Work out the finished part from the listing and answer in its coordinate system (mm). Round coordinates to 2 decimals unless told otherwise and drop trailing zeros. Loops run counter-clockwise (first coordinate to the right, second up) from the corner with the lowest first, then second, coordinate; pieces in that order, holes last. Notation, with made-up numbers: (42.25, -6) - (69.25, -6) arc R20 ccw to (69.25, 20) - close; hole circle Ø5 at (83, -21). An arc over 180 degrees is marked (long way). Return JSON: item names as keys, results as strings.
from build123d import *

# Parameters (mm, degrees)
MODEL_R         = 1
MODEL_R_2       = 1.5
EXTRUDE_1_DEPTH = 2


with BuildPart() as part:
    # Model → 凸台-拉伸1 (new body)
    with BuildSketch(Plane.XY):
        with BuildLine():
            ThreePointArc((165.794247794, 119.146851779), (174.607099306, 112.447515783), (184.890996066, 108.350087077))
            ThreePointArc((184.890996066, 108.350087077), (190.059733129, 100.139821501), (184.890996066, 91.929555925))
            ThreePointArc((184.890996066, 91.929555925), (174.607099306, 87.832127219), (165.794247794, 81.132791223))
            ThreePointArc((165.794247794, 81.132791223), (159.094911797, 72.319939711), (154.997483091, 62.036042951))
            ThreePointArc((154.997483091, 62.036042951), (146.787217515, 56.867305888), (138.576951939, 62.036042951))
            ThreePointArc((138.576951939, 62.036042951), (134.479523234, 72.319939711), (127.780187237, 81.132791223))
            ThreePointArc((127.780187237, 81.132791223), (118.967335725, 87.832127219), (108.683438965, 91.929555925))
            ThreePointArc((108.683438965, 91.929555925), (103.514701902, 100.139821501), (108.683438965, 108.350087077))
            ThreePointArc((108.683438965, 108.350087077), (118.967335725, 112.447515783), (127.780187237, 119.146851779))
            ThreePointArc((127.780187237, 119.146851779), (134.479523234, 127.959703291), (138.576951939, 138.243600051))
            ThreePointArc((138.576951939, 138.243600051), (146.787217515, 143.412337115), (154.997483091, 138.243600051))
            ThreePointArc((154.997483091, 138.243600051), (159.094911797, 127.959703291), (165.794247794, 119.146851779))
        make_face()
        with Locations((156.787217515, 110.139821501)):
            Circle(MODEL_R, mode=Mode.SUBTRACT)
        with Locations((136.787217515, 110.139821501)):
            Circle(MODEL_R, mode=Mode.SUBTRACT)
        with Locations((136.787217515, 90.139821501)):
            Circle(MODEL_R, mode=Mode.SUBTRACT)
        with Locations((156.787217515, 90.139821501)):
            Circle(MODEL_R, mode=Mode.SUBTRACT)
        with Locations((168.353974342, 100.139821501)):
            Circle(MODEL_R_2, mode=Mode.SUBTRACT)
        with Locations((146.787217515, 121.706578327)):
            Circle(MODEL_R_2, mode=Mode.SUBTRACT)
        with Locations((125.220460689, 100.139821501)):
            Circle(MODEL_R_2, mode=Mode.SUBTRACT)
        with Locations((146.787217515, 78.573064675)):
            Circle(MODEL_R_2, mode=Mode.SUBTRACT)
        with Locations((146.787217515, 126.706578327)):
            Circle(MODEL_R_2, mode=Mode.SUBTRACT)
        with Locations((120.220460689, 100.139821501)):
            Circle(MODEL_R_2, mode=Mode.SUBTRACT)
        with Locations((146.787217515, 73.573064675)):
            Circle(MODEL_R_2, mode=Mode.SUBTRACT)
        with Locations((173.353974342, 100.139821501)):
            Circle(MODEL_R_2, mode=Mode.SUBTRACT)
        with Locations((146.787217515, 118.171044401)):
            Circle(MODEL_R, mode=Mode.SUBTRACT)
        with Locations((128.755994615, 100.139821501)):
            Circle(MODEL_R, mode=Mode.SUBTRACT)
        with Locations((146.787217515, 82.108598601)):
            Circle(MODEL_R, mode=Mode.SUBTRACT)
        with Locations((164.818440415, 100.139821501)):
            Circle(MODEL_R, mode=Mode.SUBTRACT)
        with Locations((162.037217515, 115.389821501)):
            Circle(MODEL_R_2, mode=Mode.SUBTRACT)
        with Locations((131.537217515, 115.389821501)):
            Circle(MODEL_R_2, mode=Mode.SUBTRACT)
        with Locations((131.537217515, 84.889821501)):
            Circle(MODEL_R_2, mode=Mode.SUBTRACT)
        with Locations((162.037217515, 84.889821501)):
            Circle(MODEL_R_2, mode=Mode.SUBTRACT)
        with Locations((182.657217515, 100.139821501)):
            Circle(MODEL_R, mode=Mode.SUBTRACT)
        with Locations((146.787217515, 136.036864466)):
            Circle(MODEL_R, mode=Mode.SUBTRACT)
        with Locations((110.917217515, 100.139821501)):
            Circle(MODEL_R, mode=Mode.SUBTRACT)
        with Locations((146.787217515, 64.242778536)):
            Circle(MODEL_R, mode=Mode.SUBTRACT)
        with BuildLine():
            Line((152.398515146, 91.006916148), (141.004728844, 91.006916149))
            ThreePointArc((141.004728844, 91.006916149), (140.104214379, 91.379921453), (139.731209075, 92.280435918))
            ThreePointArc((139.731209075, 92.280435918), (140.104214379, 93.180950383), (141.004728844, 93.553955688))
            Line((141.004728844, 93.553955688), (152.398515146, 93.553955687))
            ThreePointArc((152.398515146, 93.553955687), (153.672034916, 92.280435917), (152.398515146, 91.006916148))
        make_face(mode=Mode.SUBTRACT)
        with BuildLine():
            Line((152.599718137, 109.199272945), (141.205931835, 109.199272945))
            ThreePointArc((141.205931835, 109.199272945), (140.30541737, 108.826267641), (139.932412066, 107.925753176))
            ThreePointArc((139.932412066, 107.925753176), (140.30541737, 107.025238711), (141.205931835, 106.652233406))
            Line((141.205931835, 106.652233406), (152.599718137, 106.652233406))
            ThreePointArc((152.599718137, 106.652233406), (153.873237907, 107.925753176), (152.599718137, 109.199272945))
        make_face(mode=Mode.SUBTRACT)
        with BuildLine():
            Line((151.898560909, 100.493374892), (147.140770906, 105.251164895))
            ThreePointArc((147.140770906, 105.251164895), (146.787217515, 105.397611504), (146.433664125, 105.251164895))
            Line((146.433664125, 105.251164895), (141.675874122, 100.493374892))
            ThreePointArc((141.675874122, 100.493374892), (141.529427512, 100.139821501), (141.675874122, 99.786268111))
            Line((141.675874122, 99.786268111), (146.433664125, 95.028478108))
            ThreePointArc((146.433664125, 95.028478108), (146.787217515, 94.882031498), (147.140770906, 95.028478108))
            Line((147.140770906, 95.028478108), (151.898560909, 99.786268111))
            ThreePointArc((151.898560909, 99.786268111), (152.045007518, 100.139821501), (151.898560909, 100.493374892))
        make_face(mode=Mode.SUBTRACT)
        with BuildLine():
            Line((137.779884988, 87.503468035), (155.779884988, 87.503468035))
            ThreePointArc((155.779884988, 87.503468035), (156.779884988, 86.503468035), (155.779884988, 85.503468035))
            Line((155.779884988, 85.503468035), (137.779884988, 85.503468035))
            ThreePointArc((137.779884988, 85.503468035), (137.072778206, 85.796361253), (136.779884988, 86.503468035))
            ThreePointArc((136.779884988, 86.503468035), (137.072778206, 87.210574816), (137.779884988, 87.503468035))
        make_face(mode=Mode.SUBTRACT)
        with BuildLine():
            Line((137.779884988, 112.776174968), (155.779884988, 112.776174968))
            ThreePointArc((155.779884988, 112.776174968), (156.779884988, 113.776174968), (155.779884988, 114.776174968))
            Line((155.779884988, 114.776174968), (137.779884988, 114.776174968))
            ThreePointArc((137.779884988, 114.776174968), (137.072778206, 114.483281749), (136.779884988, 113.776174968))
            ThreePointArc((136.779884988, 113.776174968), (137.072778206, 113.069068187), (137.779884988, 112.776174968))
        make_face(mode=Mode.SUBTRACT)
    extrude(amount=EXTRUDE_1_DEPTH)


solid = part.part
1) Determine the mould class of faces 1 (the cylindrical face through (147.325, 136.88, 0.986)), 2 (the cylindrical face through (153.873, 107.898, 0.986)), 3 (the flat face through (138, 101, 2)) for opening direction X: pulls with the +X half, pulls with the -X half, needs draft (parallel to the pull), parting line crosses it, or undercut.
Verdict:
{"face 1": "undercut", "face 2": "undercut", "face 3": "needs draft"}
2) Find the intervals of material crossed by L1, parallel to Y at x = 139.5, z = 1.4; L2, parallel to Y at x = 131, z = 0.7; L3, parallel to Y at x = 169.5, z = 0.35, in increasing order.
Verdict:
{"L1": "y = 60.51 to 85.5, 87.5 to 112.78, 114.78 to 139.77", "L2": "y = 77.51 to 83.49, 86.29 to 113.99, 116.79 to 122.77", "L3": "y = 84.42 to 99.17, 101.11 to 115.86"}
3) Section D-D (z = 1.1) is taken. Count the separate pieces of the cut face and the enclosed holes in it, and give its area (3 significant figures).
Verdict:
{"separate pieces": "1", "enclosed holes": "29", "area": "3,260 mm2"}
4) A flat-ended cylindrical pin translates along its axis: pin 1 (0.6 mm diameter, centred on x = 149, z = 1, fed in from +Y). Find the tip coordinate at first contact, or state that the pin passes through.
Verdict:
{"pin 1": "stops at y = 143.21"}
5) Section B-B (y = 104) is taken. Give the vertices of the cut face in (x, z), and give its area (3 significant figures).
Verdict:
{"outline": "(104.37, 0) - (145.18, 0) - (145.18, 2) - (104.37, 2) - close; (148.39, 0) - (189.2, 0) - (189.2, 2) - (148.39, 2) - close", "area": "163 mm2"}
6) Section A-A (x = 125.5) is taken. Give the vertices of the cut face in (y, z).
Verdict:
{"outline": "(83.25, 0) - (98.67, 0) - (98.67, 2) - (83.25, 2) - close; (101.61, 0) - (117.03, 0) - (117.03, 2) - (101.61, 2) - close"}
7) Section C-C (y = 69.5) is taken. Give the vertices of the cut face in (x, z), and give its area (3 significant figures).
Verdict:
{"outline": "(135.93, 0) - (157.64, 0) - (157.64, 2) - (135.93, 2) - close", "area": "43.4 mm2"}
